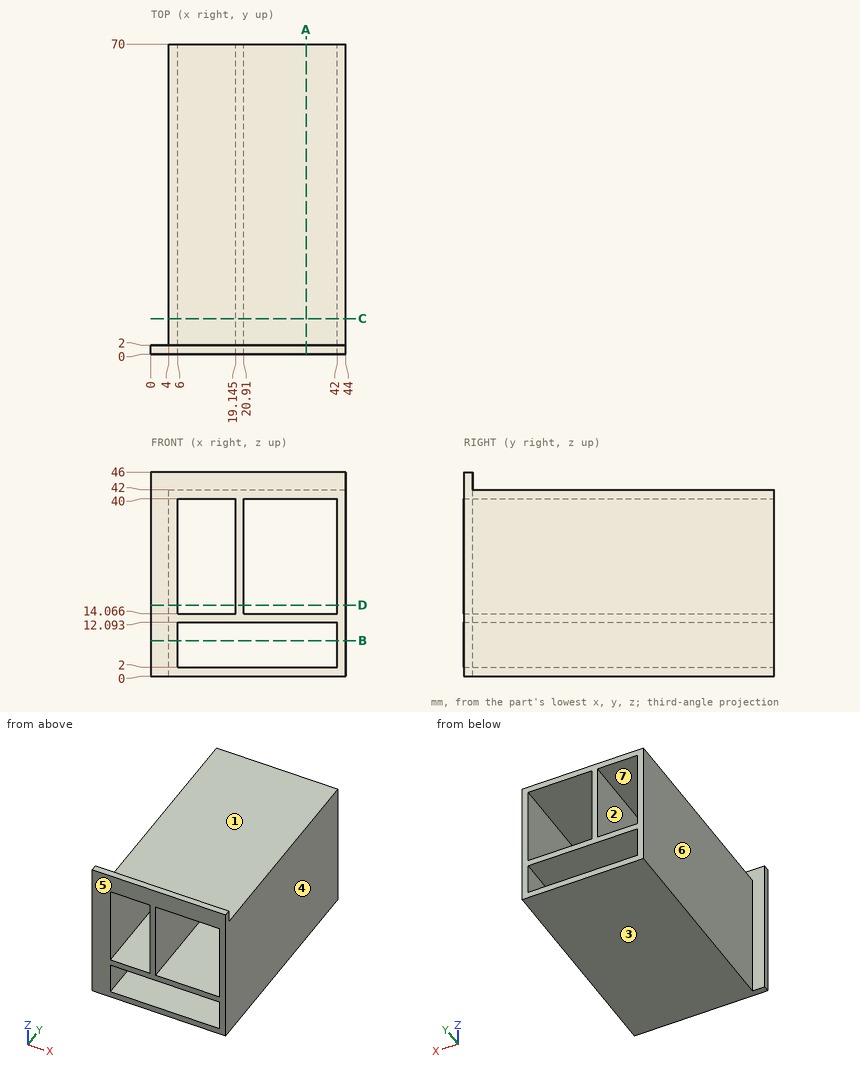
Job drawing, mm, ordinate dimensions from the low corner. One solid piece. A direction names the side the tool comes from. Round coordinates to 2 decimals unless told otherwise and drop trailing zeros. Write each loop counter-clockwise with the first axis right and the second up, starting at its lowest first coordinate (ties: lowest second). Pieces come first, ordered by that corner, then holes. Notation, with made-up numbers: (-4, 19) -> (21, 19) arc R30 cw to (21, 53) -> close; hole circle Ø5 at (47, 68). An arc over 180 degrees is marked (long way). Answer as a JSON object with one key per item and string values.
(1) Which spindle directions (+Z, -Z, +X, -X, +Y, -Y) get a long thin tool onto all of the face, cutting with end or side? Do the marked faces 1, 2 and 3. Say none if no direction does.
Reported:
{"face 1": "+Z, +X, -X, +Y", "face 2": "+Y, -Y", "face 3": "-Z, +X, -X, +Y, -Y"}
(2) Pin check, flat tips, straight feed: P1, Ø12, axis at x = 21.5, y = 40.5, coming from the +Z side; P2, Ø13, axis at y = 39.5, z = 33, coming from the -X side; P3, Ø10, axis at x = 11.5, z = 29.5, coming from the +Y side. Stop position of each tip, or through.
Reported:
{"P1": "stops at z = 42", "P2": "stops at x = 4", "P3": "passes through"}
(3) Band-saw the part on B-B, the plane z = 8. List the corners of the cut face in (x, y), then the cut area to 3 significant figures.
Reported:
{"outline": "(0, 0) -> (6, 0) -> (6, 70) -> (4, 70) -> (4, 2) -> (0, 2) -> close; (42, 0) -> (44, 0) -> (44, 70) -> (42, 70) -> close", "area": "288 mm^2"}
(4) Probe probe 1 along Z at (x, y) = (11.5, 29.5); probe 2 along X at (y, z) = (58.5, 33.5) (3 decimals); probe 3 along X at (y, z) = (44.5, 8.5). List the from-to ranges inside material, lowest first. Write a range as [from, to].
Reported:
{"probe 1": "z = [0, 2], [12.09, 14.07], [40, 42]", "probe 2": "x = [4, 6], [19.145, 20.91], [42, 44]", "probe 3": "x = [4, 6], [42, 44]"}
(5) Band-saw the part on A-A, the plane x = 35. List the corners of the cut face in (y, z), then the cut area to 3 significant figures.
Reported:
{"outline": "(0, 0) -> (70, 0) -> (70, 2) -> (0, 2) -> close; (0, 12.09) -> (70, 12.09) -> (70, 14.07) -> (0, 14.07) -> close; (0, 40) -> (70, 40) -> (70, 42) -> (2, 42) -> (2, 46) -> (0, 46) -> close", "area": "426 mm^2"}
(6) Two-plate mould, pull along X, no slides. Class the marked faces 4, 5, 6 and 7: +X half, -X half, draft (parallel to the pull), parting line (faces both ways), or undercut.
Reported:
{"face 4": "+X half", "face 5": "draft", "face 6": "-X half", "face 7": "undercut"}
(7) Band-saw the part on D-D, the plane z = 16. List the corners of the cut face in (x, y) (3 decimals).
Reported:
{"outline": "(0, 0) -> (6, 0) -> (6, 70) -> (4, 70) -> (4, 2) -> (0, 2) -> close; (19.145, 0) -> (20.91, 0) -> (20.91, 70) -> (19.145, 70) -> close; (42, 0) -> (44, 0) -> (44, 70) -> (42, 70) -> close"}
(8) Band-saw the part on C-C, the plane y = 8. List the corners of the cut face in (x, z) (3 decimals), then the cut area to 3 significant figures.
Reported:
{"outline": "(4, 0) -> (44, 0) -> (44, 42) -> (4, 42) -> close; hole (6, 2) -> (42, 2) -> (42, 12.093) -> (6, 12.093) -> close; hole (6, 14.066) -> (19.145, 14.066) -> (19.145, 40) -> (6, 40) -> close; hole (20.91, 14.066) -> (42, 14.066) -> (42, 40) -> (20.91, 40) -> close", "area": "429 mm^2"}
